```python
from build123d import *

# Parameters (mm, degrees)
SZKIC1_W                   = 70
SZKIC1_H                   = 30
ODGI_CIE_BAZOWE1_DEPTH     = 3
WYTNIJ_WYCI_GNI_CIE1_REACH = 40.197
SZKIC6_R                   = 1.5
WYTNIJ_WYCI_GNI_CIE2_REACH = 40.197
SZKIC7_R                   = 1.5
WYTNIJ_WYCI_GNI_CIE3_REACH = 40.197
SZKIC10_R                  = 1.5


# Sheet-metal steps are written as plain solids
with BuildPart() as part:
    # Szkic1 → Odgięcie bazowe1 (new body)
    with BuildSketch(Plane(origin=(0, 0, 0), x_dir=(1, 0, 0), z_dir=(0, 1, 0))):
        Rectangle(SZKIC1_W, SZKIC1_H)
    extrude(amount=-ODGI_CIE_BAZOWE1_DEPTH)

    # Szkic6 → Wytnij-wyciągnięcie1 (cut, up to next)
    with BuildSketch(Plane(origin=(0, 0, 0), x_dir=(1, 0, 0), z_dir=(0, 1, 0)), mode=Mode.PRIVATE) as wytnij_wyci_gni_cie1_sk1:
        with Locations(Location((-28, 8, 0), (0, 0, 270))):
            Circle(SZKIC6_R)
    wytnij_wyci_gni_cie1_tool1 = extrude(wytnij_wyci_gni_cie1_sk1.sketch, amount=-WYTNIJ_WYCI_GNI_CIE1_REACH, mode=Mode.PRIVATE) & part.part
    wytnij_wyci_gni_cie1 = wytnij_wyci_gni_cie1_tool1.solids().sort_by_distance((-28, 0, -8))[0]
    add(wytnij_wyci_gni_cie1, mode=Mode.SUBTRACT)

    # Lustro1: Wytnij-wyciągnięcie1 across plane
    add(wytnij_wyci_gni_cie1.mirror(Plane.XY), mode=Mode.SUBTRACT)

    # Szkic7 → Wytnij-wyciągnięcie2 (cut, up to next)
    with BuildSketch(Plane(origin=(0, 0, 0), x_dir=(1, 0, 0), z_dir=(0, 1, 0)), mode=Mode.PRIVATE) as wytnij_wyci_gni_cie2_sk1:
        with Locations(Location((28, 0, 0), (0, 0, 270))):
            Circle(SZKIC7_R)
    wytnij_wyci_gni_cie2_tool1 = extrude(wytnij_wyci_gni_cie2_sk1.sketch, amount=-WYTNIJ_WYCI_GNI_CIE2_REACH, mode=Mode.PRIVATE) & part.part
    wytnij_wyci_gni_cie2 = wytnij_wyci_gni_cie2_tool1.solids().sort_by_distance((28, 0, 0))[0]
    add(wytnij_wyci_gni_cie2, mode=Mode.SUBTRACT)

    # Szkic-szyk1: Wytnij-wyciągnięcie2 at 3 more places
    with Locations((-12.5, 0, 0), (-6.25, 0, -6.25), (-6.25, 0, 6.25)):
        add(wytnij_wyci_gni_cie2, mode=Mode.SUBTRACT)

    # Szkic10 → Wytnij-wyciągnięcie3 (cut, up to next)
    with BuildSketch(Plane(origin=(0, 0, 0), x_dir=(1, 0, 0), z_dir=(0, 1, 0)), mode=Mode.PRIVATE) as wytnij_wyci_gni_cie3_sk1:
        with Locations(Location((-4, 0, 0), (0, 0, 270))):
            Circle(SZKIC10_R)
    wytnij_wyci_gni_cie3_tool1 = extrude(wytnij_wyci_gni_cie3_sk1.sketch, amount=-WYTNIJ_WYCI_GNI_CIE3_REACH, mode=Mode.PRIVATE) & part.part
    add(wytnij_wyci_gni_cie3_tool1.solids().sort_by_distance((-4, 0, 0))[0], mode=Mode.SUBTRACT)


solid = part.part
```
Can you work these out from the model? Positions are in its coordinate system, mm. Coordinates: 2 decimals unless noted, no trailing zeros. Write each loop counter-clockwise with the first axis right and the second up, starting at its lowest first coordinate (ties: lowest second). Pieces come first, ordered by that corner, then holes. Notation, with made-up numbers: (-33, -34) - (-28, -34) arc R18 cw to (-28, -15) - close; hole circle Ø3 at (36, -30). An arc over 180 degrees is marked (long way). Return JSON: item names as keys, results as strings.
Q1. If we section it at B-B (z = 0): Please give me the cut outline in (x, y).
Computed values:
{"outline": "(-35, -3) - (-5.5, -3) - (-5.5, 0) - (-35, 0) - close; (-2.5, -3) - (14, -3) - (14, 0) - (-2.5, 0) - close; (17, -3) - (26.5, -3) - (26.5, 0) - (17, 0) - close; (29.5, -3) - (35, -3) - (35, 0) - (29.5, 0) - close"}
Q2. Please list where these lines run through material, in increasing order: L1, parallel to X at y = -1.2, z = 0; L2, parallel to X at y = -1.15, z = -8; L3, parallel to X at y = -2.3, z = 6.25. Write a range as from..to.
Computed values:
{"L1": "x = -35..-5.5, -2.5..14, 17..26.5, 29.5..35", "L2": "x = -35..-29.5, -26.5..35", "L3": "x = -35..20.25, 23.25..35"}
Q3. If we section it at A-A (x = 28): Please give me the cut outline in (y, z), then the cut area to 3 significant figures.
Computed values:
{"outline": "(-3, -15) - (0, -15) - (0, -1.5) - (-3, -1.5) - close; (-3, 1.5) - (0, 1.5) - (0, 15) - (-3, 15) - close", "area": "81.0 mm2"}
Q4. If we section it at C-C (y = -2.2): Please give me the cut outline in (x, z).
Computed values:
{"outline": "(-35, -15) - (35, -15) - (35, 15) - (-35, 15) - close; hole circle Ø3 at (-28, -8); hole circle Ø3 at (-28, 8); hole circle Ø3 at (-4, 0); hole circle Ø3 at (15.5, 0); hole circle Ø3 at (21.75, -6.25); hole circle Ø3 at (21.75, 6.25); hole circle Ø3 at (28, 0)"}
Q5. Thinking about a two-plate mould opening in Z: for faces 1 (the flat face through (0, 0, 0)), 2 (the cylindrical face through (-2.513, -1.479, -0.195)), 3 (the flat face through (0, -1, -15)), which applies, +Z half, -Z half, draft (parallel to the pull), parting line (faces both ways), or undercut?
Computed values:
{"face 1": "draft", "face 2": "undercut", "face 3": "-Z half"}
